```python
from build123d import *

# Parameters (mm, degrees)
SKETCH1_W                                       = 210
SKETCH1_H                                       = 500
BASE_FLANGE1_DEPTH                              = 10
SKETCH2_R                                       = 2.75
CUT_EXTRUDE1_DEPTH                              = 10
SKETCH3_R                                       = 3.3
CUT_EXTRUDE2_DEPTH                              = 10
SKETCH4_R                                       = 2.75
CUT_EXTRUDE3_DEPTH                              = 10
M6X1_0_TAPPED_HOLE1_D                           = 5
M6X1_0_TAPPED_HOLE1_DEPTH                       = 15
M6X1_0_TAPPED_HOLE1_CSINK_D                     = 6.05
M6X1_0_TAPPED_HOLE1_CSINK_ANGLE                 = 90
M6X1_0_TAPPED_HOLE1_TIP                         = 1.502151548
CSK_FOR_M5_FLAT_HEAD_MACHINE_SCREW1_D           = 5.5
CSK_FOR_M5_FLAT_HEAD_MACHINE_SCREW1_DEPTH       = 24.5
CSK_FOR_M5_FLAT_HEAD_MACHINE_SCREW1_CSINK_D     = 10.4
CSK_FOR_M5_FLAT_HEAD_MACHINE_SCREW1_CSINK_ANGLE = 90
CSK_FOR_M5_FLAT_HEAD_MACHINE_SCREW1_TIP         = 1.652366702
CSK_FOR_M5_FLAT_HEAD_MACHINE_SCREW2_D           = 5.5
CSK_FOR_M5_FLAT_HEAD_MACHINE_SCREW2_DEPTH       = 24.5
CSK_FOR_M5_FLAT_HEAD_MACHINE_SCREW2_CSINK_D     = 10.4
CSK_FOR_M5_FLAT_HEAD_MACHINE_SCREW2_CSINK_ANGLE = 90
CSK_FOR_M5_FLAT_HEAD_MACHINE_SCREW2_TIP         = 1.652366702


# Sheet-metal steps are written as plain solids
with BuildPart() as part:
    # Sketch1 → Base-Flange1 (new body)
    with BuildSketch(Plane.XY):
        Rectangle(SKETCH1_W, SKETCH1_H)
    extrude(amount=-BASE_FLANGE1_DEPTH)

    # Sketch2 → Cut-Extrude1 (cut)
    with BuildSketch(Plane.XY):
        with Locations((-94.75, 118)):
            Circle(SKETCH2_R)
        with Locations((-94.75, 65)):
            Circle(SKETCH2_R)
        with Locations((-54.75, 118)):
            Circle(SKETCH2_R)
        with Locations((-54.75, 65)):
            Circle(SKETCH2_R)
        with Locations((54.75, 118)):
            Circle(SKETCH2_R)
        with Locations((54.75, 65)):
            Circle(SKETCH2_R)
        with Locations((94.75, 118)):
            Circle(SKETCH2_R)
        with Locations((94.75, 65)):
            Circle(SKETCH2_R)
        with Locations((-54.75, -132)):
            Circle(SKETCH2_R)
        with Locations((-94.75, -132)):
            Circle(SKETCH2_R)
        with Locations((-94.75, -185)):
            Circle(SKETCH2_R)
        with Locations((-54.75, -185)):
            Circle(SKETCH2_R)
        with Locations((54.75, -132)):
            Circle(SKETCH2_R)
        with Locations((94.75, -132)):
            Circle(SKETCH2_R)
        with Locations((94.75, -185)):
            Circle(SKETCH2_R)
        with Locations((54.75, -185)):
            Circle(SKETCH2_R)
    extrude(amount=-CUT_EXTRUDE1_DEPTH, mode=Mode.SUBTRACT)

    # Sketch3 → Cut-Extrude2 (cut)
    with BuildSketch(Plane.XY):
        with Locations((-23, -220)):
            Circle(SKETCH3_R)
        with Locations((23, -220)):
            Circle(SKETCH3_R)
    extrude(amount=-CUT_EXTRUDE2_DEPTH, mode=Mode.SUBTRACT)

    # Sketch4 → Cut-Extrude3 (cut)
    with BuildSketch(Plane.XY):
        with Locations((12, -13.5)):
            Circle(SKETCH4_R)
        with Locations((12, -53.5)):
            Circle(SKETCH4_R)
        with Locations((-12, -53.5)):
            Circle(SKETCH4_R)
        with Locations((-12, -13.5)):
            Circle(SKETCH4_R)
    extrude(amount=-CUT_EXTRUDE3_DEPTH, mode=Mode.SUBTRACT)

    # M6x1.0 Tapped Hole1
    with Locations(Plane(origin=(0, 0, -10), x_dir=(-1, 0, 0), z_dir=(0, 0, -1))):
        with Locations((-75, 226), (-25, 226), (25, 226), (75, 226)):
            CounterSinkHole(M6X1_0_TAPPED_HOLE1_D / 2, M6X1_0_TAPPED_HOLE1_CSINK_D / 2, depth=M6X1_0_TAPPED_HOLE1_DEPTH, counter_sink_angle=M6X1_0_TAPPED_HOLE1_CSINK_ANGLE)
            with Locations((0, 0, -(M6X1_0_TAPPED_HOLE1_DEPTH + M6X1_0_TAPPED_HOLE1_TIP / 2))):  # 118° drill point
                Cone(0, M6X1_0_TAPPED_HOLE1_D / 2, M6X1_0_TAPPED_HOLE1_TIP, mode=Mode.SUBTRACT)

    # CSK for M5 Flat Head Machine Screw1
    with Locations(Plane(origin=(0, 0, 0), x_dir=(-1, 0, 0), z_dir=(0, 0, 1))):
        with Locations((-54.75, -118), (-94.75, -118), (-94.75, -65), (-54.75, -65), (54.75, -118), (94.75, -118), (54.75, -65), (94.75, -65), (-94.75, 132), (-54.75, 132), (-94.75, 185), (-54.75, 185), (54.75, 132), (54.75, 185), (94.75, 132), (94.75, 185)):
            CounterSinkHole(CSK_FOR_M5_FLAT_HEAD_MACHINE_SCREW1_D / 2, CSK_FOR_M5_FLAT_HEAD_MACHINE_SCREW1_CSINK_D / 2, depth=CSK_FOR_M5_FLAT_HEAD_MACHINE_SCREW1_DEPTH, counter_sink_angle=CSK_FOR_M5_FLAT_HEAD_MACHINE_SCREW1_CSINK_ANGLE)
            with Locations((0, 0, -(CSK_FOR_M5_FLAT_HEAD_MACHINE_SCREW1_DEPTH + CSK_FOR_M5_FLAT_HEAD_MACHINE_SCREW1_TIP / 2))):  # 118° drill point
                Cone(0, CSK_FOR_M5_FLAT_HEAD_MACHINE_SCREW1_D / 2, CSK_FOR_M5_FLAT_HEAD_MACHINE_SCREW1_TIP, mode=Mode.SUBTRACT)

    # CSK for M5 Flat Head Machine Screw2
    with Locations(Plane.XY):
        with Locations((12, -13.5), (-12, -13.5), (-12, -53.5), (12, -53.5)):
            CounterSinkHole(CSK_FOR_M5_FLAT_HEAD_MACHINE_SCREW2_D / 2, CSK_FOR_M5_FLAT_HEAD_MACHINE_SCREW2_CSINK_D / 2, depth=CSK_FOR_M5_FLAT_HEAD_MACHINE_SCREW2_DEPTH, counter_sink_angle=CSK_FOR_M5_FLAT_HEAD_MACHINE_SCREW2_CSINK_ANGLE)
            with Locations((0, 0, -(CSK_FOR_M5_FLAT_HEAD_MACHINE_SCREW2_DEPTH + CSK_FOR_M5_FLAT_HEAD_MACHINE_SCREW2_TIP / 2))):  # 118° drill point
                Cone(0, CSK_FOR_M5_FLAT_HEAD_MACHINE_SCREW2_D / 2, CSK_FOR_M5_FLAT_HEAD_MACHINE_SCREW2_TIP, mode=Mode.SUBTRACT)


solid = part.part
```
Geometry: final body of the model. Coordinates: model frame, mm. Coordinates: 2 decimals unless noted, no trailing zeros. Use CSV: the item, a comma, the result in double quotes. Start each with the question number.
1. First-contact query: P1, Ø9, axis at x = -94.75, y = -132, coming from the -Z side; P2, Ø3.5, axis at x = -12, y = -53.5, coming from the +Z side; P3, Ø9, axis at x = 54.75, y = 65, coming from the +Z side; P4, Ø7, axis at x = -54.75, y = 65, coming from the +Z side. Flat tips, straight axial feed; report the tip coordinate or a pass-through.
2. Ray query, probe 1 along Y at (x, z) = (-54.5, -7); probe 2 along X at (y, z) = (226, -1.75); probe 3 along X at (y, z) = (-132, -5.75). Return the intervals inside material, ascending.
3. Mould query, pull axis Y, two halves, no side actions, for faces 1 (the face through (-1, 250, -5)), 2 (the face through (-93.21, -134.42, -2.33)), 3 (the face through (105, -3, -5)), 4 (the face through (-11.38, -56.3, -2.33)). Classes: pulls with the +Y half, pulls with the -Y half, needs draft (parallel to the pull), parting line crosses it, or undercut.
Entries:
1,P1,"z = -10"
1,P2,"through"
1,P3,"z = -0.7"
1,P4,"z = -1.7"
2,probe 1,"-250 to -187.74, -182.26 to -134.74, -129.26 to 62.26, 67.74 to 115.26, 120.74 to 250"
2,probe 2,"-105 to -77.5, -72.5 to -27.5, -22.5 to 22.5, 27.5 to 72.5, 77.5 to 105"
2,probe 3,"-105 to -97.5, -92 to -57.5, -52 to 52, 57.5 to 92, 97.5 to 105"
3,face 1,"pulls with the +Y half"
3,face 2,"undercut"
3,face 3,"needs draft"
3,face 4,"undercut"
